Source: three-view drawing plus pictorial views. Frame: mm from the lowest corner of the part. Coordinates: 2 decimals unless noted, no trailing zeros. Write each loop counter-clockwise with the first axis right and the second up, starting at its lowest first coordinate (ties: lowest second). Pieces come first, ordered by that corner, then holes. Notation, with made-up numbers: (-29, 30) -> (17, 30) arc R10 ccw to (17, 45) -> close; hole circle Ø10 at (80, 6.25). An arc over 180 degrees is marked (long way). One line per item, written item: value.
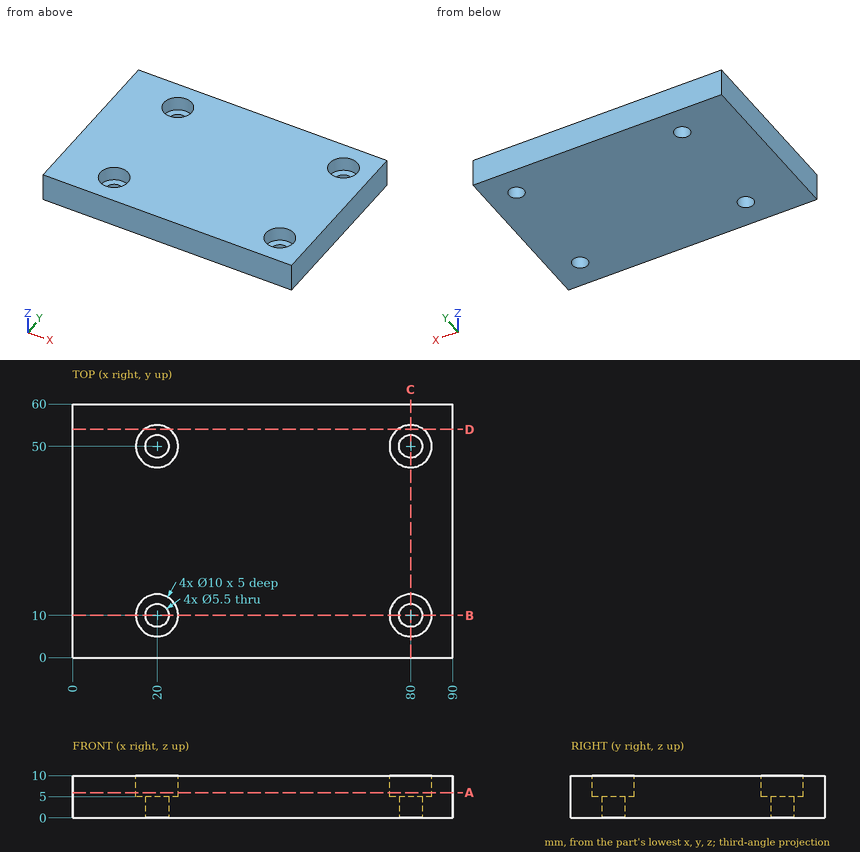
(1) Section B-B (y = 10). Return the cut outline in (x, z).
Responses:
outline: (0, 0) -> (17.25, 0) -> (17.25, 5) -> (15, 5) -> (15, 10) -> (0, 10) -> close; (22.75, 0) -> (77.25, 0) -> (77.25, 5) -> (75, 5) -> (75, 10) -> (25, 10) -> (25, 5) -> (22.75, 5) -> close; (82.75, 0) -> (90, 0) -> (90, 10) -> (85, 10) -> (85, 5) -> (82.75, 5) -> close
(2) Section A-A (z = 6). Return the cut outline in (x, y), then the cut area to 3 significant figures.
Responses:
outline: (0, 0) -> (90, 0) -> (90, 60) -> (0, 60) -> close; hole circle Ø10 at (20, 10); hole circle Ø10 at (20, 50); hole circle Ø10 at (80, 10); hole circle Ø10 at (80, 50)
area: 5,090 mm2
(3) Section C-C (x = 80). Return the cut outline in (y, z).
Responses:
outline: (0, 0) -> (7.25, 0) -> (7.25, 5) -> (5, 5) -> (5, 10) -> (0, 10) -> close; (12.75, 0) -> (47.25, 0) -> (47.25, 5) -> (45, 5) -> (45, 10) -> (15, 10) -> (15, 5) -> (12.75, 5) -> close; (52.75, 0) -> (60, 0) -> (60, 10) -> (55, 10) -> (55, 5) -> (52.75, 5) -> close
(4) First-contact query: pin 1 (5 mm diameter, centred on x = 80, y = 50, fed in from +Z); pin 2 (3 mm diameter, centred on x = 21, y = 9, fed in from +Z). Flat tips, straight axial feed; report the tip coordinate or a pass-through.
Responses:
pin 1: passes through
pin 2: stops at z = 5
(5) Line query: line 1 (Y direction, x = 80, z = 7.8); line 2 (Y direction, x = 20, z = 3.7); line 3 (X direction, y = 9, z = 6.25). Output: solid intervals per line, ascending. Write a range as [from, to].
Responses:
line 1: y = [0, 5], [15, 45], [55, 60]
line 2: y = [0, 7.25], [12.75, 47.25], [52.75, 60]
line 3: x = [0, 15.1], [24.9, 75.1], [84.9, 90]
(6) Section D-D (y = 54). Return the cut outline in (x, z).
Responses:
outline: (0, 0) -> (90, 0) -> (90, 10) -> (83, 10) -> (83, 5) -> (77, 5) -> (77, 10) -> (23, 10) -> (23, 5) -> (17, 5) -> (17, 10) -> (0, 10) -> close
